Design review of the part built by this model. Coordinates are the model's own, in mm. Coordinates: 2 decimals unless noted, no trailing zeros. Loops run counter-clockwise (first coordinate to the right, second up) from the corner with the lowest first, then second, coordinate; pieces in that order, holes last.
from build123d import *

# Parameters (mm, degrees)
SKETCH1_W               = 30
SKETCH1_H               = 25
BOSS_EXTRUDE1_DEPTH     = 1.57
CUT_EXTRUDE1_DEPTH      = 33.53789944
SKETCH2_W               = 11
SKETCH2_H               = 1.5
BOSS_EXTRUDE2_DEPTH     = 0.05
CUT_EXTRUDE2_DEPTH      = 33.53789944
CUT_EXTRUDE2_DEPTH_BACK = 33.53789944
FILLET1_R               = 1


with BuildPart() as part:
    # Sketch1 → Boss-Extrude1 (new body)
    with BuildSketch(Plane(origin=(0, 0, 0), x_dir=(1, 0, 0), z_dir=(0, 1, 0))):
        with Locations((15, 0)):
            Rectangle(SKETCH1_W, SKETCH1_H)
    extrude(amount=BOSS_EXTRUDE1_DEPTH)

    # Sketch3 → Cut-Extrude1 (cut, through all)
    with BuildSketch(Plane(origin=(0, 0, 0), x_dir=(1, 0, 0), z_dir=(0, 1, 0))):
        with BuildLine():
            Line((10.41339187, -4.139314767), (1, -4.632649731))
            Line((1, -4.632649731), (0, -5.21))
            Line((0, -5.21), (0, -2.07))
            Line((0, -2.07), (1, -2.647350269))
            Line((1, -2.647350269), (10.41339187, -3.140685233))
            ThreePointArc((10.41339187, -3.140685233), (10.887223892, -3.64), (10.41339187, -4.139314767))
        make_face()
        Polygon((11, 12.5), (1, 11.975922207), (0, 11.398571938), (0, 12.5), align=None)
        Polygon((11, -12.5), (0, -12.5), (0, -11.398571938), (1, -11.975922207), align=None)
    extrude(amount=CUT_EXTRUDE1_DEPTH, mode=Mode.SUBTRACT)

    # Sketch2 → Boss-Extrude2 (add)
    with BuildSketch(Plane(origin=(0, 0, 0), x_dir=(1, 0, 0), z_dir=(0, 1, 0))):
        with Locations((5.5, -10.1)):
            Rectangle(SKETCH2_W, SKETCH2_H)
        with Locations((5.5, -6.46)):
            Rectangle(SKETCH2_W, SKETCH2_H)
        with Locations((5.5, -0.82)):
            Rectangle(SKETCH2_W, SKETCH2_H)
        with Locations((5.5, 2.82)):
            Rectangle(SKETCH2_W, SKETCH2_H)
        with Locations((5.5, 6.46)):
            Rectangle(SKETCH2_W, SKETCH2_H)
        with Locations((5.5, 10.1)):
            Rectangle(SKETCH2_W, SKETCH2_H)
    extrude(amount=-BOSS_EXTRUDE2_DEPTH)

    # Sketch4 → Cut-Extrude2 (cut, two sides: drawn at the far end of the back side and taken through both)
    with BuildSketch(Plane(origin=(0, 0, 0), x_dir=(1, 0, 0), z_dir=(0, 1, 0)).offset(-CUT_EXTRUDE2_DEPTH_BACK)):
        with BuildLine():
            Line((0, -11.130776406), (0, -9.069223594))
            ThreePointArc((0, -9.069223594), (0.050132295, -9.287441484), (0.19047619, -9.46190032))
            ThreePointArc((0.19047619, -9.46190032), (0.5, -10.1), (0.19047619, -10.73809968))
            ThreePointArc((0.19047619, -10.73809968), (0.050132295, -10.912558516), (0, -11.130776406))
        make_face()
        with BuildLine():
            Line((0, -5.429223594), (0, -7.490776406))
            ThreePointArc((0, -7.490776406), (0.050132295, -7.272558516), (0.19047619, -7.09809968))
            ThreePointArc((0.19047619, -7.09809968), (0.5, -6.46), (0.19047619, -5.82190032))
            ThreePointArc((0.19047619, -5.82190032), (0.050132295, -5.647441484), (0, -5.429223594))
        make_face()
        with BuildLine():
            Line((0, -1.850776406), (0, 0.210776406))
            ThreePointArc((0, 0.210776406), (0.050132295, -0.007441484), (0.19047619, -0.18190032))
            ThreePointArc((0.19047619, -0.18190032), (0.5, -0.82), (0.19047619, -1.45809968))
            ThreePointArc((0.19047619, -1.45809968), (0.050132295, -1.632558516), (0, -1.850776406))
        make_face()
        with BuildLine():
            Line((0, 3.850776406), (0, 1.789223594))
            ThreePointArc((0, 1.789223594), (0.050132295, 2.007441484), (0.19047619, 2.18190032))
            ThreePointArc((0.19047619, 2.18190032), (0.5, 2.82), (0.19047619, 3.45809968))
            ThreePointArc((0.19047619, 3.45809968), (0.050132295, 3.632558516), (0, 3.850776406))
        make_face()
        with BuildLine():
            Line((0, 5.429223594), (0, 7.490776406))
            ThreePointArc((0, 7.490776406), (0.050132295, 7.272558516), (0.19047619, 7.09809968))
            ThreePointArc((0.19047619, 7.09809968), (0.5, 6.46), (0.19047619, 5.82190032))
            ThreePointArc((0.19047619, 5.82190032), (0.050132295, 5.647441484), (0, 5.429223594))
        make_face()
        with BuildLine():
            Line((0, 11.130776406), (0, 9.069223594))
            ThreePointArc((0, 9.069223594), (0.050132295, 9.287441484), (0.19047619, 9.46190032))
            ThreePointArc((0.19047619, 9.46190032), (0.5, 10.1), (0.19047619, 10.73809968))
            ThreePointArc((0.19047619, 10.73809968), (0.050132295, 10.912558516), (0, 11.130776406))
        make_face()
    extrude(amount=CUT_EXTRUDE2_DEPTH + CUT_EXTRUDE2_DEPTH_BACK, mode=Mode.SUBTRACT)

    # Fillet1
    # the kernel refuses this fillet: 1 mm, written as the material it takes off along each edge
    with BuildSketch(Plane(origin=(1, -0.600196898, -11.975922207), x_dir=(0.998629534754574, 0, -0.0523359562429405), z_dir=(0, 1, 0)), Plane(origin=(1, -0.600196898, 4.632649731), x_dir=(0.9986295347545742, 0, -0.05233595624293651), z_dir=(0, 1, 0)), Plane(origin=(1, -0.600196898, 2.647350269), x_dir=(-0.8660254037844378, 0, -0.5000000000000013), z_dir=(0, 1, 0))) as fillet1_piece_1:
        with BuildLine():
            CenterArc((FILLET1_R * 0.24007875908, -FILLET1_R), FILLET1_R, 90, 27)
            Line((-FILLET1_R * 0.213911740659, -FILLET1_R * 0.108993475812), (-FILLET1_R * 0.222991550654, -FILLET1_R * 0.0911733453279))
            Line((-FILLET1_R * 0.222991550654, -FILLET1_R * 0.0911733453279), (-FILLET1_R * 0.0048015751816, FILLET1_R * 0.02))
            Line((-FILLET1_R * 0.0048015751816, FILLET1_R * 0.02), (FILLET1_R * 0.24007875908, FILLET1_R * 0.02))
            Line((FILLET1_R * 0.24007875908, FILLET1_R * 0.02), (FILLET1_R * 0.24007875908, 0))
        make_face()
    extrude(amount=2.770393795, mode=Mode.SUBTRACT)
    with BuildSketch(Plane(origin=(0, -1.266133532, -11.398571938), x_dir=(0.8660254037844373, 0, -0.5000000000000024), z_dir=(0, 1, 0))) as fillet1_piece_2:
        with BuildLine():
            CenterArc((0.506453413, -1), FILLET1_R, 90, 39.818010975)
            Line((-0.133897766, -0.231917733), (-0.146704789, -0.216556088))
            ThreePointArc((-0.146704789, -0.216556088), (-0.084269391, -0.105958867), (-0.017320508, 0.01))
            Line((-0.017320508, 0.01), (0, 0.02))
            Line((0, 0.02), (0.506453413, 0.02))
            Line((0.506453413, 0.02), (0.506453413, 0))
        make_face()
    extrude(amount=4.102267063, mode=Mode.SUBTRACT)
    with BuildSketch(Plane(origin=(0, -1.191538155, 5.21), x_dir=(0.8660254037844375, 0, -0.500000000000002), z_dir=(0, 1, 0))) as fillet1_piece_3:
        with BuildLine():
            CenterArc((0.476615262, -1), FILLET1_R, 90, 35.889723461)
            Line((-0.109611797, -0.189853201), (-0.121336338, -0.173650265))
            ThreePointArc((-0.121336338, -0.173650265), (-0.072126406, -0.084926601), (-0.017320508, 0.01))
            Line((-0.017320508, 0.01), (0, 0.02))
            Line((0, 0.02), (0.476615262, 0.02))
            Line((0.476615262, 0.02), (0.476615262, 0))
        make_face()
    extrude(amount=3.953076309, mode=Mode.SUBTRACT)
    with BuildSketch(Plane(origin=(0, -1.191538155, 2.07), x_dir=(0, 0, -1), z_dir=(0, 1, 0))) as fillet1_piece_4:
        with BuildLine():
            CenterArc((0.627717773, -0.912760925), FILLET1_R, 114.110276539, 35.889723461)
            Line((-0.238307631, -0.412760925), (-0.255628139, -0.402760925))
            Line((-0.255628139, -0.402760925), (-0.017320508, 0.01))
            Line((-0.017320508, 0.01), (0, 0.02))
            ThreePointArc((0, 0.02), (0.109611797, 0.02), (0.21105371, 0.018255218))
            Line((0.21105371, 0.018255218), (0.219223594, 0))
        make_face()
    extrude(amount=3.953076309, mode=Mode.SUBTRACT)
    with BuildSketch(Plane(origin=(0, -1.266133532, 11.398571938), x_dir=(3.4310526757958135e-12, 0, -1.0), z_dir=(0, 1, 0))) as fillet1_piece_5:
        with BuildLine():
            CenterArc((0.612798697, -0.938601521), FILLET1_R, 110.181989025, 39.818010975)
            Line((-0.253226706, -0.438601521), (-0.270547214, -0.428601521))
            Line((-0.270547214, -0.428601521), (-0.017320508, 0.01))
            Line((-0.017320508, 0.01), (0, 0.02))
            ThreePointArc((0, 0.02), (0.133897766, 0.02), (0.260895468, 0.01877203))
            Line((0.260895468, 0.01877203), (0.267795532, 0))
        make_face()
    extrude(amount=4.102267063, mode=Mode.SUBTRACT)
    with BuildSketch(Plane(origin=(1, -0.600196898, 11.975922207), x_dir=(0.998629534754574, 0, 0.0523359562429404), z_dir=(0, 1, 0))) as fillet1_piece_6:
        with BuildLine():
            CenterArc((FILLET1_R * 0.24007875908, FILLET1_R), FILLET1_R, 243, 27)
            Line((-FILLET1_R * 0.213911740659, FILLET1_R * 0.108993475812), (-FILLET1_R * 0.222991550654, FILLET1_R * 0.0911733453279))
            Line((-FILLET1_R * 0.222991550654, FILLET1_R * 0.0911733453279), (-FILLET1_R * 0.0048015751816, -FILLET1_R * 0.02))
            Line((-FILLET1_R * 0.0048015751816, -FILLET1_R * 0.02), (FILLET1_R * 0.24007875908, -FILLET1_R * 0.02))
            Line((FILLET1_R * 0.24007875908, -FILLET1_R * 0.02), (FILLET1_R * 0.24007875908, 0))
        make_face()
    extrude(amount=2.770393795, mode=Mode.SUBTRACT)
    with BuildSketch(Plane(origin=(11, -0.065464804, -12.5), x_dir=(-0.998629534754574, 0, 0.05233595624294029), z_dir=(0, 1, 0)), Plane(origin=(11, -0.065464804, 12.5), x_dir=(1, 0, 0), z_dir=(0, 1, 0))) as fillet1_piece_7:
        with BuildLine():
            CenterArc((FILLET1_R * 0.0261859215692, FILLET1_R), FILLET1_R, 267, 3)
            Line((-FILLET1_R * 0.0261500346738, FILLET1_R * 0.00137046524543), (-FILLET1_R * 0.0271967537986, -FILLET1_R * 0.0186021254497))
            Line((-FILLET1_R * 0.0271967537986, -FILLET1_R * 0.0186021254497), (-FILLET1_R * 0.000523718431384, -FILLET1_R * 0.02))
            Line((-FILLET1_R * 0.000523718431384, -FILLET1_R * 0.02), (FILLET1_R * 0.0261859215692, -FILLET1_R * 0.02))
            Line((FILLET1_R * 0.0261859215692, -FILLET1_R * 0.02), (FILLET1_R * 0.0261859215692, 0))
        make_face()
    extrude(amount=1.700929608, mode=Mode.SUBTRACT)


solid = part.part
Q1. Take a section at B-B, the plane z = 3.64. Write out the cut boundary in (x, y).
Q2. Clearance check with a flat-ended pin moving along its axis: pin 1 Ø12.5 at (x, z) = (21.5, -4.5) entering from -Y. State where the tip first meets the part, or that it passes through.
Q3. Take a section at C-C, the plane x = 24. Write out the cut boundary in (y, z), then the cut area to 4 significant figures.
Q4. For line 1 (Y direction, x = 15.5, z = 1.75); line 2 (Z direction, x = 5.5, y = 0.4); line 3 (X direction, y = 0.5, z = 6.5), list the stretches that pass through material, from the lowest coordinate up.
Q5. The part is to be moulded in two halves that separate along Z. For faces 1 (the flat face through (6.175, 0.774, -12.247)), 2 (the flat face through (5, -0.05, 1)), 3 (the cylindrical face through (0.5, 0.7, 6.5)), say which applies: pulls with the +Z half, pulls with the -Z half, needs draft (parallel to the pull), parting line crosses it, or undercut.
Entries:
1. outline: (10.89, 0) - (30, 0) - (30, 1.57) - (10.89, 1.57) - close
2. pin 1: stops at y = 0
3. outline: (0, -12.5) - (1.57, -12.5) - (1.57, 12.5) - (0, 12.5) - close
3. area: 39.25 mm2
4. line 1: y = 0 to 1.57
4. line 2: z = -12.21 to 2.88, 4.4 to 12.21
4. line 3: x = 0.5 to 30
5. face 1: pulls with the -Z half
5. face 2: needs draft
5. face 3: undercut
